Autodesk Inventor part; units mm, degrees
ref_plane "Work Plane1" through (65, 45, -30.5) normal (0, 0, -1) x (-1, 0, 0)
ref_plane "YZ Plane" through (0, 0, 0) normal (1, 0, 0) x (0, 1, 0)
ref_plane "XZ Plane" through (0, 0, 0) normal (0, 1, 0) x (-1, 0, 0)
sketch "Sketch1" plane through (0, 0, 0) normal (0, 0, 1) x (1, 0, 0)
  line L0 (-31, -31) -> (31, -31)
  line L1 (31, -31) -> (31, 31)
  line L2 (31, 31) -> (-31, 31)
  line L3 (-31, 31) -> (-31, -31)
  line L4 (-31, -31) -> (31, 31) construction
  line L5 (31, -31) -> (-31, 31) construction
  line L6 (-33, 33) -> (33, 33)
  line L7 (33, 33) -> (33, -33)
  line L8 (33, -33) -> (-33, -33)
  line L9 (-33, -33) -> (-33, 33)
  point P0 (0, 0)
  dimension "d0" = 62
  dimension "d1" = 62
  dimension "d2" = 2
extrude "Extrusion1" add sketch "Sketch1" along normal blind 2 contours L3 L2 L1 L0 | L6 L7 L8 L9
extrude "Extrusion2" add sketch "Sketch1" against normal blind 12
sketch "Sketch2" plane through (-33, 33, 2) normal (0, 1, 0) x (1, 0, 0)
  line L0 (13, 3) -> (53, 3)
  line L1 (53, 3) -> (53, 0)
  line L2 (53, 0) -> (13, 0)
  line L3 (13, 0) -> (13, 3)
  line L4 (0, 14) -> (0, 0)
  line L5 (0, 14) -> (66, 14)
  point P0 (33, 2)
  dimension "d7" = 40
  dimension "d8" = 3
  dimension "d9" = 13
  dimension "d10" = 11
extrude "Extrusion3" add sketch "Sketch2" along normal blind 12
sketch "Sketch3" plane through (20, 33, -1) normal (0, 0, -1) x (-1, 0, 0)
  line L0 (40, 12) -> (0, 12)
  line L1 (40, 0) -> (40, 12)
  line L2 (0, 12) -> (40, 12)
  line L3 (40, 12) -> (40, 9)
  line L4 (40, 9) -> (0, 9)
  line L5 (0, 9) -> (0, 12)
  point P0 (20, -33)
  dimension "d13" = 3
extrude "Extrusion4" add sketch "Sketch3" along normal blind 80
sketch "Sketch4" plane through (-20, 42, -1) normal (0, -1, 0) x (1, 0, 0)
  line L0 (30.5, -63) -> (9.5, -63)
  line L1 (9.5, -63) -> (9.5, -22)
  line L2 (9.5, -22) -> (30.5, -22)
  line L3 (30.5, -22) -> (30.5, -63)
  line L4 (40, 3) -> (40, -80)
  line L5 (0, 3) -> (40, 3)
  point P0 (20, 1)
  dimension "d16" = 21
  dimension "d17" = 41
  dimension "d18" = 9.5
  dimension "d19" = 25
extrude "Extrusion5" cut sketch "Sketch4" against normal blind 80
sketch "Sketch5" plane through (-20, 42, -1) normal (0, -1, 0) x (1, 0, 0)
  line L0 (30.5, -63) -> (9.5, -63)
  line L1 (30.5, -63) -> (9.5, -63)
  line L2 (9.5, -63) -> (9.5, -70)
  line L3 (9.5, -70) -> (30.5, -70)
  line L4 (30.5, -70) -> (30.5, -63)
  circle A0 centre (15, -66.75) radius 2.25
  line L5 (30.5, -22) -> (30.5, -63)
  line L6 (30.5, -22) -> (9.5, -22)
  line L7 (9.5, -22) -> (9.5, -15)
  line L8 (9.5, -15) -> (30.5, -15)
  line L9 (30.5, -15) -> (30.5, -22)
  circle A1 centre (25, -18.25) radius 2.25
  point P0 (20, 1)
  point P1 (15.4717, -69.81)
  point P2 (14.5283, -69.81)
  point P3 (24.5283, -15.19)
  point P4 (25.4717, -15.19)
  dimension "d22" = 7
  dimension "d23" = 4.5
  dimension "d24" = 3.75
  dimension "d25" = 5.5
  dimension "d26" = 7
  dimension "d27" = 4.5
  dimension "d28" = 5.5
  dimension "d29" = 3.75
extrude "Extrusion6" cut sketch "Sketch5" against normal blind 80 contours A0 | A1
sketch "Sketch6" plane through (-33, -33, 2) normal (0, -1, 0) x (1, 0, 0)
  line L0 (0, 0) -> (66, 0)
  line L1 (66, -14) -> (0, -14)
  line L2 (0, 0) -> (66, 0)
  line L3 (66, 0) -> (66, -14)
  line L4 (66, -14) -> (0, -14)
  line L5 (0, -14) -> (0, 0)
  point P0 (33, -2)
extrude "Extrusion7" cut sketch "Sketch6" against normal up to surface (75 mm away)
sketch "Sketch7" plane through (-20, 42, -81) normal (0, -1, 0) x (1, 0, 0)
  line L0 (40, 83) -> (40, 0)
  line L1 (40, 0) -> (85, 0)
  line L2 (85, 0) -> (85, 83)
  line L3 (85, 83) -> (40, 83)
  line L4 (40, 83) -> (40, 0)
  line L5 (85, 33) -> (40, 33)
  point P0 (20, 81)
  point P1 (40, 33)
  dimension "d34" = 45
  dimension "d35" = 83
  dimension "d36" = 50
extrude "Extrusion8" add sketch "Sketch7" against normal up to surface (3 mm away) contours L3 L2 L5 L0
sketch "Sketch8" plane through (-20, 42, -81) normal (0, -1, 0) x (1, 0, 0)
  line L0 (0, 83) -> (85, 83)
  line L1 (85, 83) -> (85, 0)
  line L2 (85, 0) -> (0, 0)
  line L3 (0, 0) -> (0, 83)
  line L4 (85, 7) -> (0, 7)
  line L5 (85, 33) -> (85, 83)
  line L6 (-12.2623, 85.093) -> (0, 83)
  line L7 (0, 83) -> (-11.5686, 87.0435)
  line L8 (-11.5686, 87.0435) -> (85, 70.5603)
  line L9 (0, 83) -> (100, 83)
  line L10 (100, 83) -> (100, 68)
  line L11 (100, 68) -> (0, 68)
  line L12 (0, 68) -> (0, 83)
  point P0 (20, 81)
  point P1 (0, 73.8499)
  point P2 (27.25, 61.75)
  point P3 (27.25, 61.75)
  point P4 (25.55, 64.81)
  point P5 (0, 68)
  point P6 (85, 68)
  dimension "d40" = 83
  dimension "d41" = 7
  dimension "d43" = 15
extrude "Extrusion9" cut sketch "Sketch8" against normal blind 10 contours L0 L8 L1 L11 L3 | L0 L1 L8 | L4 L1 L2 L3
sketch "Sketch9" plane through (20, 42, -48) normal (0, -1, 0) x (1, 0, 0)
  line L0 (45, 0) -> (45, 35)
  line L1 (0, 0) -> (45, 0)
  line L2 (45, 35) -> (42, 35)
  line L3 (42, 35) -> (42, 0)
  line L4 (42, 0) -> (45, 0)
  line L5 (45, 0) -> (45, 35)
  point P0 (-20, 48)
  dimension "d46" = 3
extrude "Extrusion10" add sketch "Sketch9" along normal blind 100
sketch "Sketch10" plane through (65, 45, -13) normal (1, 0, 0) x (0, 0, -1)
  circle A0 centre (18, -56.25) radius 2.125
  circle A1 centre (18, -93) radius 2.125
  circle A2 centre (18, -74.625) radius 6.45
  line L0 (20.093, -55.8824) -> (22.589, -70.0925)
  line L1 (15.9065, -55.8857) -> (13.439, -70.0643)
  line L2 (20.0935, -93.3643) -> (22.561, -79.1857)
  line L3 (15.8877, -93.2317) -> (13.411, -79.1575)
  line L4 (18, -56.25) -> (18, -74.625)
  line L5 (18, -74.625) -> (18, -93)
  line L6 (35, 0) -> (35, -103)
  line L7 (35, -103) -> (0, -103)
  point P0 (-13, -45)
  dimension "d49" = 4.25
  dimension "d50" = 4.25
  dimension "d51" = 12.9
  dimension "d52" = 9.15
  dimension "d53" = 9.15
  dimension "d54" = 41
  dimension "d57" = 17
  dimension "d58" = 10
extrude "Extrusion11" cut sketch "Sketch10" against normal blind 2.5
sketch "Sketch11" plane through (65, 45, -13) normal (1, 0, 0) x (0, 0, -1)
  line L0 (35, -3) -> (35, -103)
  line L1 (0, 0) -> (0, -103)
  line L2 (35, -103) -> (0, -103)
  line L3 (0, -103) -> (0, 0)
  line L4 (0, 0) -> (35, 0)
  line L5 (35, 0) -> (35, -103)
  line L6 (35, -40) -> (0, -40)
  point P0 (-13, -45)
  dimension "d59" = 40
extrude "Extrusion12" cut sketch "Sketch11" against normal blind 10 contours L0 L2 L1 L6
sketch "Sketch12" plane through (65, 45, -48) normal (0, 0, -1) x (-1, 0, 0)
  line L0 (45, -3) -> (3, -3)
  line L1 (3, -3) -> (45, -3)
  line L2 (45, -3) -> (45, -13)
  line L3 (45, -13) -> (3, -13)
  line L4 (3, -13) -> (3, -3)
  line L5 (3, -13) -> (45, -3)
  point P0 (65, -45)
  dimension "d62" = 42
  dimension "d63" = 10
extrude "Extrusion13" add sketch "Sketch12" against normal blind 2 contours L5 L4 L0
ref_plane "Work Plane1" through (65, 45, -30.5) normal (0, 0, -1) x (-1, 0, 0)
mirror "Mirror1" about plane through (65, 45, -30.5) normal (0, 0, -1) of "Extrusion13"
sketch "Sketch13" plane through (65, 45, -13) normal (1, 0, 0) x (0, 0, -1)
  circle A0 centre (17.382, -23) radius 5.5
  circle A1 centre (17.382, -23) radius 6.45
  circle A2 centre (-0.993, -23) radius 2.125
  circle A3 centre (35.757, -23) radius 2.125
  line L0 (-1.339, -20.9034) -> (12.6745, -18.5907)
  line L1 (-1.3774, -25.0899) -> (13.0021, -27.7348)
  line L2 (36.1038, -20.9035) -> (22.084, -18.5848)
  line L3 (36.1414, -25.0899) -> (21.762, -27.7348)
  line L4 (17.382, -23) -> (35.757, -23)
  line L5 (17.382, -23) -> (-0.993, -23)
  circle A4 centre (3.207, -27.4) radius 1.15
  circle A5 centre (31.557, -18.6) radius 1.15
  line L6 (0, -40) -> (35, -40)
  line L7 (-0.993, -23) -> (35.757, -23)
  circle A6 centre (31.557, -27.4) radius 1.15
  circle A7 centre (3.207, -18.6) radius 1.15
  circle A8 centre (12.982, -37.175) radius 1.15
  circle A9 centre (21.782, -37.175) radius 1.15
  circle A10 centre (21.782, -8.825) radius 1.15
  circle A11 centre (12.982, -8.825) radius 1.15
  circle A12 centre (31.557, -27.4) radius 1.15
  circle A13 centre (31.557, -18.6) radius 1.15
  circle A14 centre (3.207, -18.6) radius 1.15
  circle A15 centre (3.207, -27.4) radius 1.15
  circle A16 centre (21.782, -8.825) radius 1.15
  circle A17 centre (12.982, -8.825) radius 1.15
  circle A18 centre (12.982, -37.175) radius 1.15
  circle A19 centre (21.782, -37.175) radius 1.15
  point P0 (-13, -45)
  point P1 (17.5, -40)
  dimension "d66" = 12.9
  dimension "d67" = 4.25
  dimension "d68" = 4.25
  dimension "d69" = 9.15
  dimension "d70" = 9.15
  dimension "d71" = 41
  dimension "d72" = 18.375
  dimension "d73" = 2.3
  dimension "d74" = 4.4
  dimension "d75" = 4.2
  dimension "d76" = 2.3
  dimension "d77" = 4.4
  dimension "d78" = 4.2
  dimension "d79" = 17
  dimension "d86" = 360
extrude "Extrusion14" cut sketch "Sketch13" against normal blind 10 contours A4 | A5
extrude "Extrusion15" cut sketch "Sketch13" against normal blind 10 contours A6 | A7
extrude "Extrusion16" cut sketch "Sketch13" against normal blind 10 contours A8 | A9 | A10 | A11
extrude "Extrusion17" cut sketch "Sketch13" against normal blind 10 contours L4 L5 A0 | A0 L5 L4
properties part number "pan_base_holder_second"
Input: part model. Units: mm. Frame: model coordinates. A direction names the side the tool comes from. Round coordinates to 2 decimals unless told otherwise and drop trailing zeros. Loops run counter-clockwise (first coordinate to the right, second up) from the corner with the lowest first, then second, coordinate; pieces in that order, holes last.
1) Section query A-A on z = -41. Return the cut outline in (x, y), plus the area to 3 significant figures.
Ans:
outline: (-20, 42) - (-10.5, 42) - (-10.5, 45) - (-20, 45) - close; (10.5, 42) - (62, 42) - (62, 5) - (65, 5) - (65, 45) - (10.5, 45) - close
area: 303 mm2
2) Material intervals for line 1 (Z direction, x = -5, y = 42.9); line 2 (Z direction, x = 64, y = 17); line 3 (X direction, y = 42.5, z = -19), sorted ascending.
Ans:
line 1: z = -74 to -70, -65.5 to -64, -23 to -13
line 2: z = -48 to -45.54, -43.58 to -32.67, -28.09 to -17.19, -15.23 to -13
line 3: x = -20 to 2.76, 7.24 to 65
3) Section query C-C on x = 5. Return the cut outline in (y, z).
Ans:
outline: (42, -74) - (45, -74) - (45, -64) - (42, -64) - close; (42, -23) - (45, -23) - (45, -21.5) - (42, -21.5) - close; (42, -17) - (45, -17) - (45, -13) - (42, -13) - close
4) Pin query (flat end, axial travel): pin 1 (14.5 mm diameter, centred on y = 22, z = -30.382, fed in from -X); pin 2 (0.9 mm diameter, centred on y = 43.5, z = -61, fed in from +X); pin 3 (1.5 mm diameter, centred on x = 30.5, y = 39.5, fed in from -Z); pin 4 (1.4 mm diameter, centred on y = 7.825, z = -34.782, fed in from +X). Return the tip coordinate at first contact, or that it passes through.
Ans:
pin 1: stops at x = 62
pin 2: stops at x = 20
pin 3: stops at z = -48
pin 4: passes through
5) Set-up query: faces 4 (the cylindrical face through (63.52, 18.38, -43.71)), 5 (the flat face through (0, 43, -64)), 6 (the flat face through (20, 42, -36)), 7 (the flat face through (41, 37, -47)), 8 (the flat face through (20, 43, -61)). Return all of +Z, -Z, +X, -X, +Y, -Y with unobstructed straight access to the full face (end or side cutting, diameter ignored); none if empty.
Ans:
face 4: +X, -X
face 5: +Y, -Y
face 6: -X, -Y
face 7: +Z, -Z, -X, -Y
face 8: -Z, +X, +Y, -Y
6) Section query B-B on y = 23.5. Return the cut outline in (x, z), plus the area to 3 significant figures.
Ans:
outline: (62, -48) - (65, -48) - (65, -35.67) - (62, -35.67) - close; (62, -25.09) - (65, -25.09) - (65, -13) - (62, -13) - close
area: 73.3 mm2
7) Section query D-D on y = 40.5. Return the cut outline in (x, z), plus the area to 3 significant figures.
Ans:
outline: (26.3, -48) - (65, -48) - (65, -13) - (26.3, -13) - (26.3, -15) - (62, -15) - (62, -46) - (26.3, -46) - close
area: 248 mm2
8) Pull-direction query (Z, two-part tool) for faces 1 (the flat face through (0, 43, -74)), 2 (the cylindrical face through (63.521, 17.945, -17.304)), 3 (the flat face through (64, 5, -31)); classes: released by +Z, released by -Z, zero draft, split by the parting line, or undercut.
Ans:
face 1: released by -Z
face 2: undercut
face 3: zero draft
